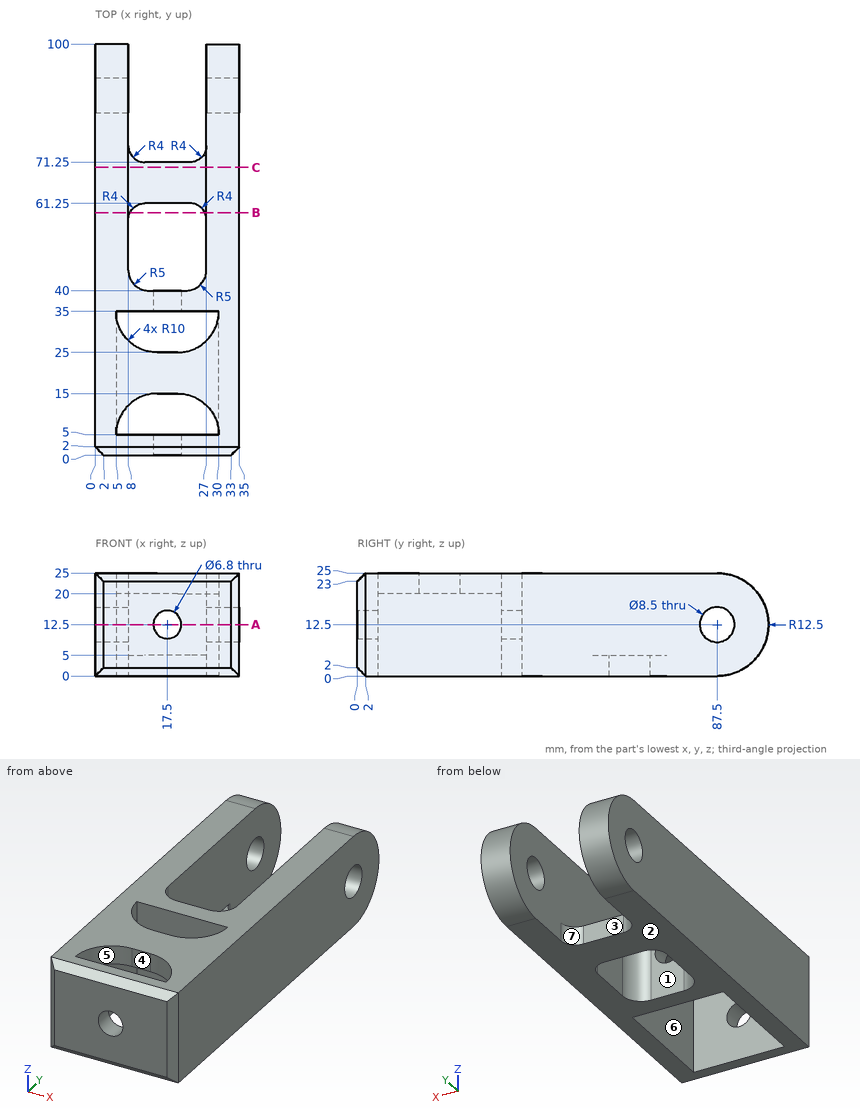
For this review, use the dimensioned drawing (mm, ordinates from the lowest corner) and the shaded views. A direction names the side the tool comes from. Round coordinates to 2 decimals unless told otherwise and drop trailing zeros. Write each loop counter-clockwise with the first axis right and the second up, starting at its lowest first coordinate (ties: lowest second). Pieces come first, ordered by that corner, then holes. Notation, with made-up numbers: (-38, -15.75) - (-15, -15.75) arc R11 ccw to (-15, -7.75) - close; hole circle Ø5 at (-13.5, 25.5). An arc over 180 degrees is marked (long way). Answer as CSV lines item,"result". Start each with the question number.
(1) We need section B-B on y = 59. State the section outline as (x, z) points.
(2) For pin 1 Ø7 at (x, z) = (19, 11.5) entering from +Y (3 decimals); pin 2 Ø12.5 at (x, y) = (20.5, 25) entering from -Z; pin 3 Ø2.5 at (x, z) = (16.5, 2) entering from +Y, all flat-tipped, find the tip position at first contact; note any pin that passes through.
(3) To check wall thickness, follow line 1 (X direction, y = 90, z = 20.5); line 2 (X direction, y = 3.75, z = 12.5); line 3 (Y direction, x = 29.5, z = 12.5). State the ranges of each line that lie inside material, in increasing order.
(4) Draft analysis for pull direction Y (two halves, no side actions). For the marked faces 1, 2, 3 and 4, state which applies: pulls with the +Y half, pulls with the -Y half, needs draft (parallel to the pull), parting line crosses it, or undercut.
(5) For the marked faces 5, 6 and 7, list the 3-axis set-ups (+Z, -Z, +X, -X, +Y, -Y) from which the entire face can be reached by the end or side of a thin tool; tool diameter is ignored.
(6) We need section A-A on z = 12.5. Give the number of separate pieces and of enclosed holes in the cut face, plus the area to 3 significant figures.
(7) We need section C-C on y = 70. State the section outline as (x, z) points, plus the area to 3 significant figures.
Worked answers:
1,outline,"(0, 0) - (8.4, 0) - (8.4, 5) - (8, 5) - (8, 25) - (0, 25) - close; (26.6, 0) - (35, 0) - (35, 25) - (27, 25) - (27, 5) - (26.6, 5) - close"
2,pin 1,"y = 40.025"
2,pin 2,"z = 20"
2,pin 3,"y = 71.25"
3,line 1,"0 to 8, 27 to 35"
3,line 2,"0 to 14.1, 20.9 to 35"
3,line 3,"0 to 5, 35 to 83.25, 91.75 to 100"
4,face 1,"undercut"
4,face 2,"needs draft"
4,face 3,"pulls with the +Y half"
4,face 4,"undercut"
5,face 5,"+Z, -Z"
5,face 6,"-Z"
5,face 7,"+Z, -Z, +Y"
6,separate pieces,"4"
6,enclosed holes,"0"
6,area,"1,410 mm²"
7,outline,"(0, 0) - (35, 0) - (35, 25) - (27, 25) - (27, 5) - (8, 5) - (8, 25) - (0, 25) - close"
7,area,"495 mm²"
